CAD build for the part. Positions are in the model's coordinates, mm. A direction names the side the tool comes from. Coordinates: 2 decimals unless noted, no trailing zeros. Write each loop counter-clockwise with the first axis right and the second up, starting at its lowest first coordinate (ties: lowest second). Pieces come first, ordered by that corner, then holes.
Autodesk Inventor part; units mm, degrees
ref_plane "YZ Plane" through (0, 0, 0) normal (1, 0, 0) x (0, 1, 0)
ref_plane "XZ Plane" through (0, 0, 0) normal (0, 1, 0) x (-1, 0, 0)
ref_plane "XY Plane" through (0, 0, 0) normal (0, 0, 1) x (1, 0, 0)
sketch "Sketch1" plane through (0, 0, 0) normal (0, 0, 1) x (1, 0, 0)
  circle A0 centre (0, 0) radius 2.1
  arc A1 (0, 3.5) -> (0, -3.5) centre (0, 0) ccw
  line L0 (0, 3.5) -> (136, 3.5)
  line L1 (136, 3.5) -> (136, -3.5)
  line L2 (136, -3.5) -> (0, -3.5)
  dimension "d0" = 4.2
  dimension "d1" = 7
  dimension "d2" = 136
extrude "Extrusion1" add sketch "Sketch1" along normal blind 4
sketch "Sketch2" plane through (0, 3.5, 0) normal (0, 1, 0) x (1, 0, 0)
  line L0 (136, 0) -> (0, 0)
  line L1 (0, 0) -> (0, -4)
  line L2 (136, -4) -> (0, -4)
  line L3 (136, 0) -> (136, -4)
  line L4 (134, -2.75) -> (126, -2.75)
  line L5 (126, -2.75) -> (126, -1.25)
  line L6 (126, -1.25) -> (134, -1.25)
  line L7 (134, -1.25) -> (134, -2.75)
  line L8 (134, -2.75) -> (126, -1.25) construction
  line L9 (126, -2.75) -> (134, -1.25) construction
  point P0 (130, -2)
  dimension "d5" = 8
  dimension "d6" = 1.5
  dimension "d7" = 130
extrude "Extrusion2" cut sketch "Sketch2" against normal blind 6 contours L4 L5 L6 L7
fillet "Fillet1" radius 2 2 edges at (136, 0, 4) (136, 0, 0)
sketch "Sketch3" plane through (0, 0, 4) normal (0, 0, 1) x (1, 0, 0)
  line L0 (134, 3.5) -> (134, -3.5)
  line L1 (134, 3.5) -> (0, 3.5)
  arc A0 (0, 3.5) -> (0, -3.5) centre (0, 0) ccw
  line L2 (0, -3.5) -> (134, -3.5)
  circle A1 centre (0, 0) radius 2.1
  line L3 (126, 3.5) -> (126, -2.5)
  line L4 (17, 5.5) -> (117, 5.5)
  line L5 (117, 5.5) -> (117, 1.5)
  line L6 (117, 1.5) -> (17, 1.5)
  line L7 (17, 1.5) -> (17, 5.5)
  line L8 (134, 3.5) -> (0, 3.5)
  line L9 (17, 5.5) -> (117, 1.5) construction
  line L10 (117, 5.5) -> (17, 1.5) construction
  point P0 (67, 3.5)
  dimension "d11" = 100
  dimension "d12" = 4
extrude "Extrusion3" cut sketch "Sketch3" against normal blind 6 contours L5 L6 L7 L1 | L1 L7 L4 L5
fillet "Fillet2" radius 1 4 edges at (17, 1.5, 2) (17, 3.5, 2) (117, 3.5, 2) (117, 1.5, 2)
properties part number "Potentiometer Pushrod"
Item 1: Flat gauge pins, fed straight in: pin 1 Ø0.8 at (y, z) = (1.5, 1.5) entering from +X; pin 2 Ø2 at (x, z) = (71.5, 0.5) entering from +Y; pin 3 Ø2 at (y, z) = (-2.5, 1.5) entering from -X. Where does each tip first touch, or does it go through?
Item 2: Saw through at B-B, the plane x = 114. Write the cut outline in (y, z), and give its area (3 significant figures).
Item 3: Saw through at A-A, the plane y = 0. State how many separate pieces and enclosed holes the cut face has, and give its area (3 significant figures).
Item 4: Which spindle directions (+Z, -Z, +X, -X, +Y, -Y) get a long thin tool onto all of the face, cutting with end or side? Do faces 1 (the flat face through (68, 1.5, 2)), 2 (the flat face through (130, 1, 2.75)), 3 (the flat face through (8, 3.5, 2)). Say none if no direction does.
Item 5: Wall check: line 1 along X through (y, z) = (-0.25, 2.05); line 2 along Y through (x, z) = (0, 1.25); line 3 along X through (y, z) = (0.5, 2.2). Give the ranges that are in metal, low to high.
Item 6: Two-plate mould, pull along Y, no slides. Class faces 4 (the flat face through (69, -3.5, 2)), 5 (the cylindrical face through (2.003, -0.631, 1.972)), 6 (the flat face through (130, 1, 1.25)): +Y half, -Y half, draft (parallel to the pull), parting line (faces both ways), or undercut.
Working result:
1. pin 1: stops at x = 136
1. pin 2: stops at y = 1.5
1. pin 3: stops at x = -3.16
2. outline: (-3.5, 0) - (1.5, 0) - (1.5, 4) - (-3.5, 4) - close
2. area: 20.0 mm2
3. separate pieces: 2
3. enclosed holes: 1
3. area: 527 mm2
4. face 1: +Z, -Z, +Y
4. face 2: +Y
4. face 3: +Z, -Z, +X, -X, +Y
5. line 1: x = -3.49 to -2.09, 2.09 to 126, 134 to 136
5. line 2: y = -3.5 to -2.1, 2.1 to 3.5
5. line 3: x = -3.46 to -2.04, 2.04 to 126, 134 to 135.99
6. face 4: -Y half
6. face 5: undercut
6. face 6: draft
